Verification items for this drawing (mm, ordinates from the low corner). A direction names the side the tool comes from. Coordinates: 2 decimals unless noted, no trailing zeros. Loops run counter-clockwise (first coordinate to the right, second up) from the corner with the lowest first, then second, coordinate; pieces in that order, holes last. Notation, with made-up numbers: (78.5, 36.25) -> (87.5, 36.25) arc R18 ccw to (87.5, 49.25) -> close; hole circle Ø4 at (42.5, 45.25). An arc over 180 degrees is marked (long way). Write item = value, one per line.
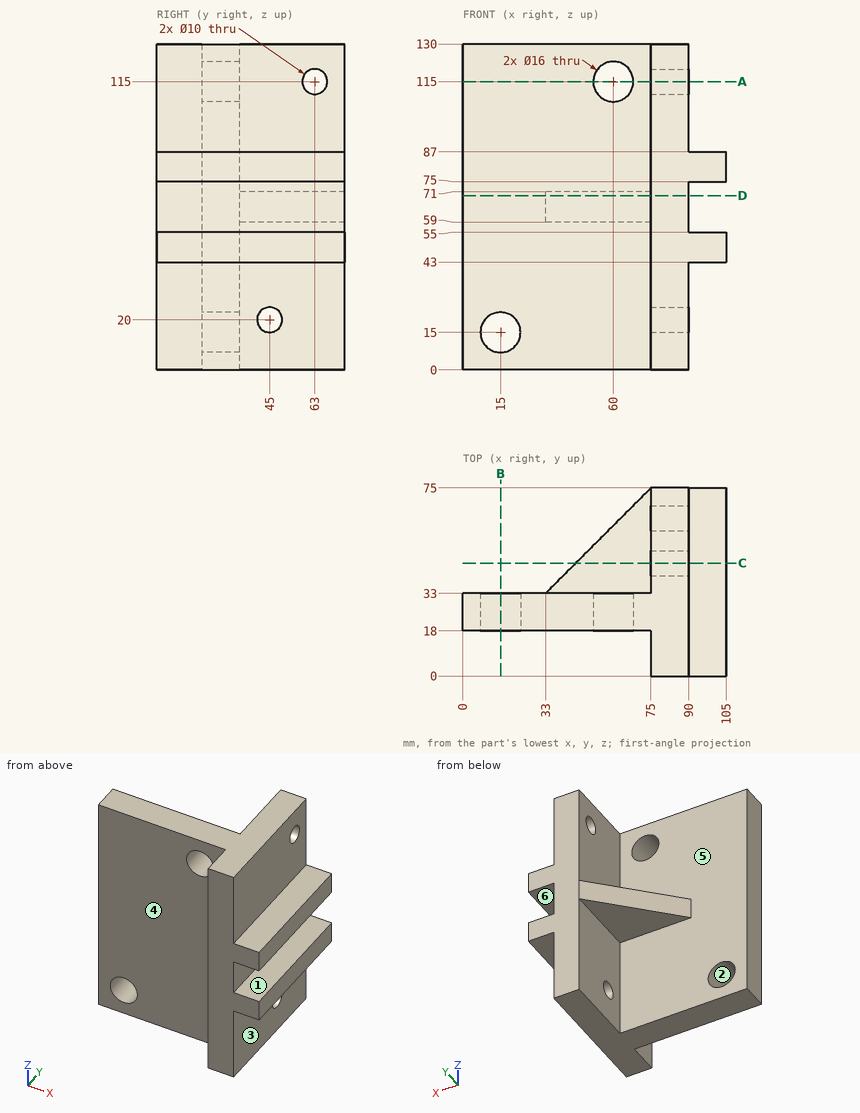
1) Depth check by flat-ended pin: pin 1 Ø12 at (x, y) = (45.5, 50.5) entering from -Z; pin 2 Ø8 at (y, z) = (51.5, 33.5) entering from +X; pin 3 Ø8 at (x, y) = (58.5, 49.5) entering from +Z; pin 4 Ø8 at (y, z) = (63, 115) entering from -X. Enter the tip coordinate at first touch or a pass-through.
Ans:
pin_1 = 59
pin_2 = 90
pin_3 = 71
pin_4 = through
2) Sectioned sample at C-C, the plane y = 45. Record the cut outline in (x, z).
Ans:
outline = (45, 59) -> (75, 59) -> (75, 25) -> (90, 25) -> (90, 43) -> (105, 43) -> (105, 55) -> (90, 55) -> (90, 75) -> (105, 75) -> (105, 87) -> (90, 87) -> (90, 130) -> (75, 130) -> (75, 71) -> (45, 71) -> close; (75, 0) -> (90, 0) -> (90, 15) -> (75, 15) -> close
3) Tool access check on the marked faces 4, 5 and 6. Record the directions out of +Z, -Z, +X, -X, +Y, -Y that give a thin tool (end or side, any length) a straight path to the whole face; none if there is none.
Ans:
face_4 = +Z, -Z, -X, -Y
face_5 = -X, +Y
face_6 = +X, +Y, -Y
4) Material ranges on line 1 (X direction, y = 27.5, z = 15); line 2 (Z direction, x = 79, y = 63); line 3 (Y direction, x = 80.25, z = 115), recorded low to high.
Ans:
line_1 = 0 to 7, 23 to 90
line_2 = 0 to 110, 120 to 130
line_3 = 0 to 58, 68 to 75
5) Sectioned sample at D-D, the plane z = 69.5. Record the cut outline in (x, y).
Ans:
outline = (0, 18) -> (75, 18) -> (75, 0) -> (90, 0) -> (90, 75) -> (75, 75) -> (33, 33) -> (0, 33) -> close
6) Sectioned sample at B-B, the plane x = 15. Record the cut outline in (y, z).
Ans:
outline = (18, 0) -> (33, 0) -> (33, 7) -> (18, 7) -> close; (18, 23) -> (33, 23) -> (33, 130) -> (18, 130) -> close
7) Sectioned sample at A-A, the plane z = 115. Record the cut outline in (x, y), plus the area to 3 significant figures.
Ans:
outline = (0, 18) -> (52, 18) -> (52, 33) -> (0, 33) -> close; (68, 18) -> (75, 18) -> (75, 0) -> (90, 0) -> (90, 58) -> (75, 58) -> (75, 33) -> (68, 33) -> close; (75, 68) -> (90, 68) -> (90, 75) -> (75, 75) -> close
area = 1,860 mm2
8) Release check for a two-part mould opening along X. For the marked faces 1, 2 and 3 record: pulls with the +X half, pulls with the -X half, needs draft (parallel to the pull), parting line crosses it, or undercut.
Ans:
face_1 = needs draft
face_2 = undercut
face_3 = pulls with the +X half
